For this review, use the dimensioned drawing (mm, ordinates from the lowest corner) and the shaded views. A direction names the side the tool comes from. Give positions to 0.01 mm unless a question says otherwise; leave off trailing zeros. Write each loop counter-clockwise with the first axis right and the second up, starting at its lowest first coordinate (ties: lowest second). Pieces come first, ordered by that corner, then holes. Notation, with made-up numbers: (-3.75, -13) -> (5.25, -13) arc R14 cw to (5.25, 10) -> close; hole circle Ø11 at (-8.5, 81.25). An arc over 180 degrees is marked (long way). Answer as CSV lines item,"result".
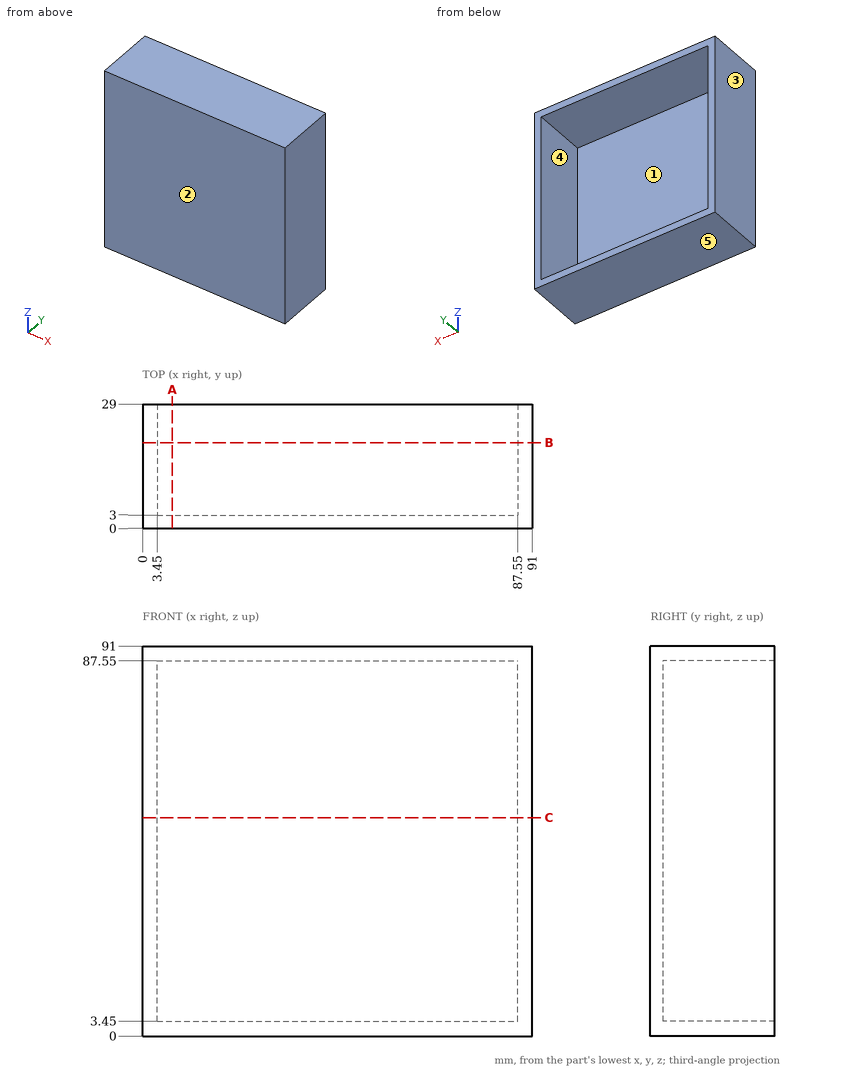
Q1. Add section C-C (z = 51). Write out the cut boundary in (x, y).
Answer block:
outline,"(0, 0) -> (91, 0) -> (91, 29) -> (87.55, 29) -> (87.55, 3) -> (3.45, 3) -> (3.45, 29) -> (0, 29) -> close"
Q2. For the marked faces 4 and 5, list the 3-axis set-ups (+Z, -Z, +X, -X, +Y, -Y) from which the entire face can be reached by the end or side of a thin tool; tool diameter is ignored.
Answer block:
face 4,"+Y"
face 5,"-Z, +X, -X, +Y, -Y"
Q3. To check wall thickness, follow probe 1 along X at (y, z) = (7.75, 30); probe 2 along Y at (x, z) = (27, 29.5). State the ranges of each line that lie inside material, in increasing order. Write a range as [from, to].
Answer block:
probe 1,"x = [0, 3.45], [87.55, 91]"
probe 2,"y = [0, 3]"
Q4. Add section B-B (y = 20). Write out the cut boundary in (x, z).
Answer block:
outline,"(0, 0) -> (91, 0) -> (91, 91) -> (0, 91) -> close; hole (3.45, 3.45) -> (87.55, 3.45) -> (87.55, 87.55) -> (3.45, 87.55) -> close"
Q5. Draft analysis for pull direction X (two halves, no side actions). For the marked faces 1, 2 and 3, state which applies: released by +X, released by -X, zero draft, split by the parting line, or undercut.
Answer block:
face 1,"undercut"
face 2,"zero draft"
face 3,"released by -X"
Q6. Add section A-A (x = 7). Write out the cut boundary in (y, z).
Answer block:
outline,"(0, 0) -> (29, 0) -> (29, 3.45) -> (3, 3.45) -> (3, 87.55) -> (29, 87.55) -> (29, 91) -> (0, 91) -> close"
Q7. Clearance check with a flat-ended pin moving along its axis: pin 1 (3 mm diameter, centred on x = 77.5, z = 37, fed in from +Y). State where the tip first meets the part, or that it passes through.
Answer block:
pin 1,"stops at y = 3"
